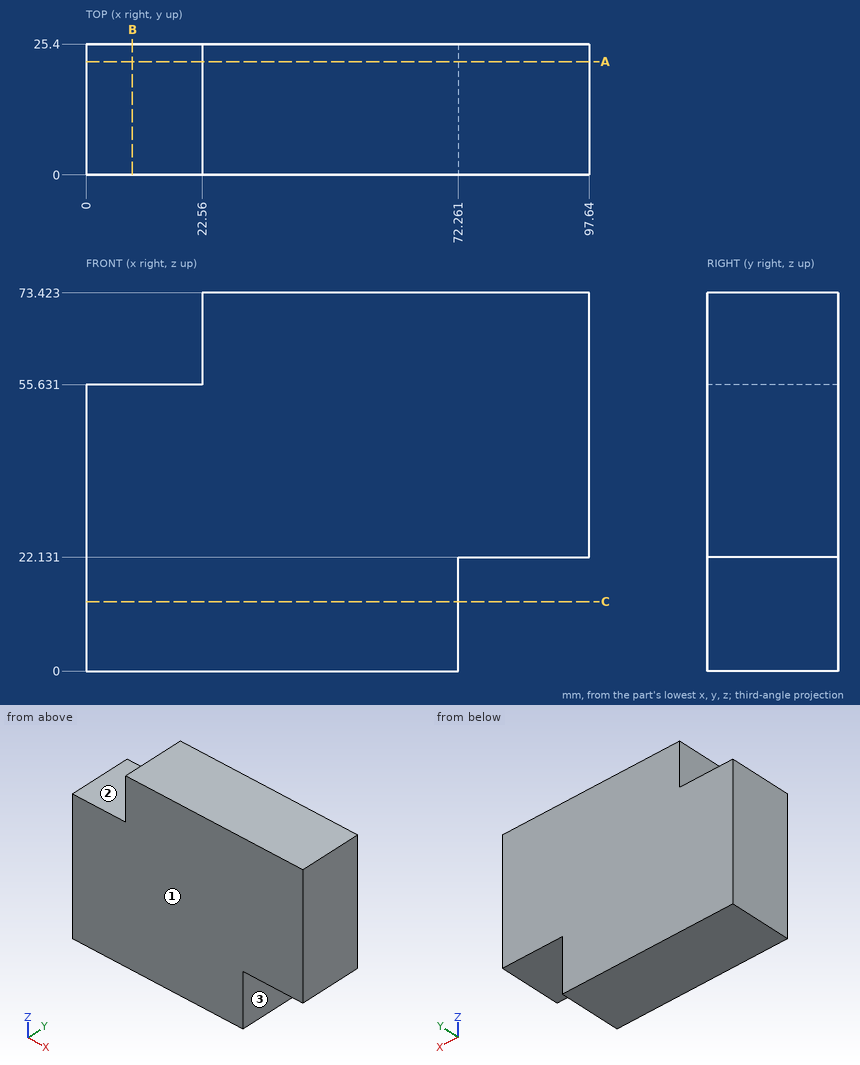
Here's the drawing with two shaded views (mm, measured from the low corner). I have some questions. A direction names the side the tool comes from. Coordinates: 2 decimals unless noted, no trailing zeros. Write each loop counter-clockwise with the first axis right and the second up, starting at its lowest first coordinate (ties: lowest second). Pieces come first, ordered by that corner, then holes. Notation, with made-up numbers: (-9, -6.5) -> (30, -6.5) arc R19 ccw to (30, 25.5) -> close; hole circle Ø6 at (-1.5, 23.25). An arc over 180 degrees is marked (long way). Write item = value, one per line. Start each with the question number.
(1) I want a section at A-A (y = 22). Please give me the cut outline in (x, z).
(2) I want a section at C-C (z = 13.5). Please give me the cut outline in (x, y).
(3) Which directions (+Z, -Z, +X, -X, +Y, -Y) give clear straight access to the entire face, cutting with the end or side of a thin tool? Please do the marked faces 1, 2 and 3.
(4) Will these pins go through, and if not, where does the flat tip stop? pin 1 (4 mm diameter, centred on x = 83.5, y = 14.5, fed in from -Z); pin 2 (11.5 mm diameter, centred on x = 13.5, y = 18.5, fed in from +Z).
(5) I want a section at B-B (x = 9). Please give me the cut outline in (y, z).
(6) I need wall thicknesses on line 1 (Z direction, x = 75, y = 20.25); line 2 (X direction, y = 9.5, z = 9.5); line 3 (Z direction, x = 11, y = 15). Which ranges of each line are inside material? Lowest first, please. Write a range as [from, to].
Result set:
q1.outline = (0, 0) -> (72.26, 0) -> (72.26, 22.13) -> (97.64, 22.13) -> (97.64, 73.42) -> (22.56, 73.42) -> (22.56, 55.63) -> (0, 55.63) -> close
q2.outline = (0, 0) -> (72.26, 0) -> (72.26, 25.4) -> (0, 25.4) -> close
q3.face_1 = +Z, -Z, +X, -X, -Y
q3.face_2 = +Z, -X, +Y, -Y
q3.face_3 = -Z, +X, +Y, -Y
q4.pin_1 = 22.13
q4.pin_2 = 55.63
q5.outline = (0, 0) -> (25.4, 0) -> (25.4, 55.63) -> (0, 55.63) -> close
q6.line_1 = [22.13, 73.42]
q6.line_2 = [0, 72.26]
q6.line_3 = [0, 55.63]
